Model file for the job. Use its own axes, mm. A direction names the side the tool comes from. Round coordinates to 2 decimals unless told otherwise and drop trailing zeros. Loops run counter-clockwise (first coordinate to the right, second up) from the corner with the lowest first, then second, coordinate; pieces in that order, holes last. Notation, with made-up numbers: M 63,79.5 L 101,79.5 A23 cw 101,92.5 Z; hole C 9.5,8.25 d3. An arc over 180 degrees is marked long. Answer in a Markdown table with one row per item.
from build123d import *

# Parameters (mm, degrees)
F0_W     = 60
F0_H     = 50
F0_R     = 10
F1_DEPTH = 52
F3_D     = 7
F3_DEPTH = 18
F3_TIP   = 2.1030121666


with BuildPart() as f1:
    # F0 (on Top) → F1 (new body, symmetric)
    with BuildSketch(Plane.XY):
        Rectangle(F0_W, F0_H)
        Circle(F0_R, mode=Mode.SUBTRACT)
    extrude(amount=F1_DEPTH, both=True)

    # F3
    with Locations(Plane.XZ.offset(25)):
        with Locations((22.5, 27.5), (-22.5, -27.5)):
            Hole(F3_D / 2, depth=F3_DEPTH)
            with Locations((0, 0, -(F3_DEPTH + F3_TIP / 2))):  # 118° drill point
                Cone(0, F3_D / 2, F3_TIP, mode=Mode.SUBTRACT)


solid = f1.part
1. Wall check: probe 1 along Z at (x, y) = (22.5, -20); probe 2 along X at (y, z) = (-15.25, 27.5); probe 3 along Y at (x, z) = (-3, 20). Give the ranges that are in metal, low to high.
Verdict:
| item | result |
|---|---|
| probe 1 | z = -52 to 24, 31 to 52 |
| probe 2 | x = -30 to 19, 26 to 30 |
| probe 3 | y = -25 to -9.54, 9.54 to 25 |
2. Saw through at A-A (x = -6). Write the cut outline in (y, z).
Verdict:
| item | result |
|---|---|
| outline | M -25,-52 L -8,-52 L -8,52 L -25,52 Z; M 8,-52 L 25,-52 L 25,52 L 8,52 Z |
3. Saw through at B-B (y = 0). Write the cut outline in (x, z), and give its area (3 significant figures).
Verdict:
| item | result |
|---|---|
| outline | M -30,-52 L -10,-52 L -10,52 L -30,52 Z; M 10,-52 L 30,-52 L 30,52 L 10,52 Z |
| area | 4,160 mm² |
4. Saw through at C-C (z = 19). Write the cut outline in (x, y).
Verdict:
| item | result |
|---|---|
| outline | M -30,-25 L 30,-25 L 30,25 L -30,25 Z; hole C 0,0 d20 |
5. Tool access for faces 4 (the flat face through (30, 0, 1)), 5 (the cylindrical face through (-22.04, -15.87, -24.03)): list every direction of +Z, -Z, +X, -X, +Y, -Y with a clear straight run to the whole face (end or side of a thin tool).
Verdict:
| item | result |
|---|---|
| face 4 | +Z, -Z, +X, +Y, -Y |
| face 5 | -Y |
6. Mould opens along X. For faces 1 (the flat face through (0, 11, 52)), 2 (the flat face through (-30, 0, 1)), 3 (the cylindrical face through (22.96, -15.87, 30.97)) say: +X half, -X half, draft (parallel to the pull), parting line (faces both ways), or undercut.
Verdict:
| item | result |
|---|---|
| face 1 | draft |
| face 2 | -X half |
| face 3 | undercut |
